Geometry: final body of the model. Coordinates: model frame, mm. Face numbers are marked on the shaded views. A direction names the side the tool comes from. Coordinates: 2 decimals unless noted, no trailing zeros. Write each loop counter-clockwise with the first axis right and the second up, starting at its lowest first coordinate (ties: lowest second). Pieces come first, ordered by that corner, then holes. Notation, with made-up numbers: (53, -33) - (109, -33) arc R26 ccw to (109, -4) - close; hole circle Ø8 at (-29.5, -15.5). An arc over 180 degrees is marked (long way). Put each result on its own line as item: value.
```python
from build123d import *

# Parameters (mm, degrees)
BOSS_EXTRUDE1_DEPTH = 2
SKETCH2_W           = 2
SKETCH2_H           = 7
BOSS_EXTRUDE2_DEPTH = 2.7
CUT_EXTRUDE1_DEPTH  = 1
CUT_EXTRUDE2_REACH  = 12.656
SKETCH4_R           = 0.59
SKETCH5_W           = 3.9
SKETCH5_H           = 4.7
BOSS_EXTRUDE3_DEPTH = 1
FILLET1_R           = 1


with BuildPart() as part:
    # Sketch1 → Boss-Extrude1 (new body)
    with BuildSketch(Plane(origin=(0, 0, 0), x_dir=(1, 0, 0), z_dir=(0, 1, 0))):
        Polygon((2.075, -3.5), (2.825, -3.5), (3.825, -3.5), (4.825, -3.5), (4.825, 3.5), (3.825, 3.5), (2.825, 3.5), (2.075, 3.5), (-2.075, 3.5), (-4.075, 3.5), (-4.075, -3.5), (-2.075, -3.5), align=None)
    extrude(amount=BOSS_EXTRUDE1_DEPTH)

    # Sketch2 → Boss-Extrude2 (add)
    with BuildSketch(Plane(origin=(0, 2, 0), x_dir=(1, 0, 0), z_dir=(0, 1, 0))):
        with Locations((-3.075, 0)):
            Rectangle(SKETCH2_W, SKETCH2_H)
        with Locations((3.825, 0)):
            Rectangle(SKETCH2_W, SKETCH2_H)
    extrude(amount=BOSS_EXTRUDE2_DEPTH)

    # Sketch3 → Cut-Extrude1 (cut)
    with BuildSketch(Plane.ZY.offset(-2.825)):
        Polygon((-0.095299462, 3.7), (-0.672649731, 4.7), (-1.827350269, 4.7), (-2.404700538, 3.7), (-1.827350269, 2.7), (-0.672649731, 2.7), align=None)
        Polygon((3.154700538, 3.7), (2.577350269, 4.7), (1.422649731, 4.7), (0.845299462, 3.7), (1.422649731, 2.7), (2.577350269, 2.7), align=None)
    extrude(amount=-CUT_EXTRUDE1_DEPTH, mode=Mode.SUBTRACT)

    # Sketch4 → Cut-Extrude2 (cut, up to next)
    with BuildSketch(Plane(origin=(4.825, 0, 0), x_dir=(0, 0, -1), z_dir=(1, 0, 0)), mode=Mode.PRIVATE) as cut_extrude2_sk1:
        with Locations((-2, 3.7)):
            Circle(SKETCH4_R)
    cut_extrude2_tool1 = extrude(cut_extrude2_sk1.sketch, amount=-CUT_EXTRUDE2_REACH, mode=Mode.PRIVATE) & part.part
    # Sketch4 → Cut-Extrude2 (cut, up to next)
    with BuildSketch(Plane(origin=(4.825, 0, 0), x_dir=(0, 0, -1), z_dir=(1, 0, 0)), mode=Mode.PRIVATE) as cut_extrude2_sk2:
        with Locations((1.25, 3.7)):
            Circle(SKETCH4_R)
    cut_extrude2_tool2 = extrude(cut_extrude2_sk2.sketch, amount=-CUT_EXTRUDE2_REACH, mode=Mode.PRIVATE) & part.part
    add(cut_extrude2_tool1.solids().sort_by_distance((4.825, 3.7, 2))[0], mode=Mode.SUBTRACT)
    add(cut_extrude2_tool2.solids().sort_by_distance((4.825, 3.7, -1.25))[0], mode=Mode.SUBTRACT)

    # Sketch5 → Boss-Extrude3 (add)
    with BuildSketch(Plane(origin=(0, 0, -3.5), x_dir=(-1, 0, 0), z_dir=(0, 0, -1))):
        with Locations((-2.875, 2.35)):
            Rectangle(SKETCH5_W, SKETCH5_H)
    extrude(amount=BOSS_EXTRUDE3_DEPTH)

    # Fillet1
    fillet1_edges = [part.edges().sort_by_distance(p)[0] for p in [
        (0.925, 1, -3.5),
    ]]
    fillet(fillet1_edges, radius=FILLET1_R - 0.0001)  # a hair under: the kernel refuses the full size


solid = part.part
```
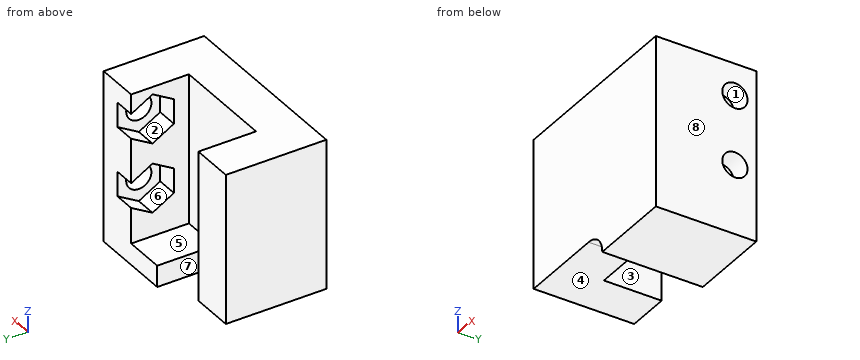
1. Section query B-B (z = 2). Return loops of the section in (x, y) (3 decimals), then the cut area to 3 significant figures.
Answer below:
outline: (-4.075, 0) - (4.825, 0) - (4.825, 3.11) - (3.825, 3.11) - (3.825, 2.7) - (2.825, 2.7) - (2.825, 2) - (-2.075, 2) - (-2.075, 4.7) - (-4.075, 4.7) - close; (3.825, 4.29) - (4.825, 4.29) - (4.825, 4.7) - (3.825, 4.7) - close
area: 25.4 mm²
2. Mould query, pull axis X, two halves, no side actions, for the marked faces 6, 7 and 8. Classes: +X half, -X half, draft (parallel to the pull), parting line (faces both ways), or undercut.
Answer below:
face 6: undercut
face 7: -X half
face 8: +X half
3. Pin query (flat end, axial travel): pin 1 Ø1.1 at (y, z) = (3.7, 2) entering from +X (3 decimals); pin 2 Ø1.2 at (x, y) = (-2.5, 1.5) entering from -Z; pin 3 Ø1.5 at (x, z) = (-0.5, -0.5) entering from +Y. Return the tip coordinate at first contact, or that it passes through.
Answer below:
pin 1: stops at x = -2.075
pin 2: stops at z = -3.5
pin 3: stops at y = 2
4. Section query D-D (x = 3). Return loops of the section in (y, z), then the cut area to 3 significant figures.
Answer below:
outline: (0, -4.5) - (4.7, -4.5) - (4.7, -1.83) - (3.7, -2.4) - (2.7, -1.83) - (2.7, -0.67) - (3.7, -0.1) - (4.7, -0.67) - (4.7, 1.42) - (3.7, 0.85) - (2.7, 1.42) - (2.7, 2.58) - (3.7, 3.15) - (4.7, 2.58) - (4.7, 3.5) - (0, 3.5) - close
area: 30.7 mm²
5. Ray query, probe 1 along Y at (x, z) = (4.5, 2); probe 2 along X at (y, z) = (2.2, -0.25) (3 decimals); probe 3 along Y at (x, z) = (-0.5, 1.25). Return the intervals inside material, ascending. Write a range as from..to.
Answer below:
probe 1: y = 0..3.11, 4.29..4.7
probe 2: x = -4.075..-2.075, 2.825..4.825
probe 3: y = 0..2
6. Section query C-C (y = 3.9). Return loops of the section in (x, z) (3 decimals), then the cut area to 3 significant figures.
Answer below:
outline: (-4.075, -3.5) - (-2.075, -3.5) - (-2.075, 3.5) - (-4.075, 3.5) - close; (0.925, -4.5) - (4.825, -4.5) - (4.825, -1.805) - (3.825, -1.805) - (3.825, -2.289) - (2.825, -2.289) - (2.825, -3.5) - (0.925, -3.5) - close; (2.825, -0.211) - (3.825, -0.211) - (3.825, -0.695) - (4.825, -0.695) - (4.825, 1.445) - (3.825, 1.445) - (3.825, 0.961) - (2.825, 0.961) - close; (2.825, 3.039) - (3.825, 3.039) - (3.825, 2.555) - (4.825, 2.555) - (4.825, 3.5) - (2.825, 3.5) - close
area: 25.5 mm²
7. Section query A-A (y = 2.5). Return loops of the section in (x, z) (3 decimals).
Answer below:
outline: (-4.075, -3.5) - (-2.075, -3.5) - (-2.075, 3.5) - (-4.075, 3.5) - close; (0.925, -4.5) - (4.825, -4.5) - (4.825, 3.5) - (2.825, 3.5) - (2.825, -3.5) - (0.925, -3.5) - close
8. Set-up query: the marked faces 1, 2, 3, 4 and 5. Return all of +Z, -Z, +X, -X, +Y, -Y with unobstructed straight access to the full face (end or side cutting, diameter ignored); none if empty.
Answer below:
face 1: +X
face 2: none
face 3: +Z, -Z, +Y
face 4: -Z, -X, +Y, -Y
face 5: +Z, +Y
